Can you work these out from the model? Positions are in its coordinate system, mm. Face numbers are marked on the shaded views. A direction names the side the tool comes from. Give positions to 0.01 mm unless a question says otherwise; leave off trailing zeros. Order: outer loops, then holes, each group sorted by start corner. A loop starts at its lowest first (then second) coordinate and runs counter-clockwise, first axis right, second up. Notation, with made-up numbers: (-24.5, 67) -> (11.5, 67) arc R9 ccw to (11.5, 82) -> close; hole circle Ø5 at (-16.75, 70). An arc over 180 degrees is marked (long way). Answer as a JSON object with one key per item and string values.
```python
from build123d import *

# Parameters (mm, degrees)
F1_DEPTH       = 22.5
F3_DEPTH       = 10
F5_D           = 10
F5_CBORE_D     = 20
F5_CBORE_DEPTH = 5


with BuildPart() as f1:
    # F0 (on Front) → F1 (new body, symmetric)
    with BuildSketch(Plane.XZ):
        Polygon((0, 45), (0, 0), (65, 0), (65, 10), (55, 10), (55, 45), align=None)
    extrude(amount=F1_DEPTH, both=True)

    # F2 (on face) → F3 (cut)
    with BuildSketch(Plane.YZ.offset(55)):
        Polygon((-22.5, 45), (-22.5, 30), (22.5, 45), align=None)
    extrude(amount=-F3_DEPTH, mode=Mode.SUBTRACT)

    # F5 (through all)
    with Locations(Plane.XY.offset(45)):
        with Locations((22.5, 0)):
            CounterBoreHole(F5_D / 2, F5_CBORE_D / 2, F5_CBORE_DEPTH)


solid = f1.part
```
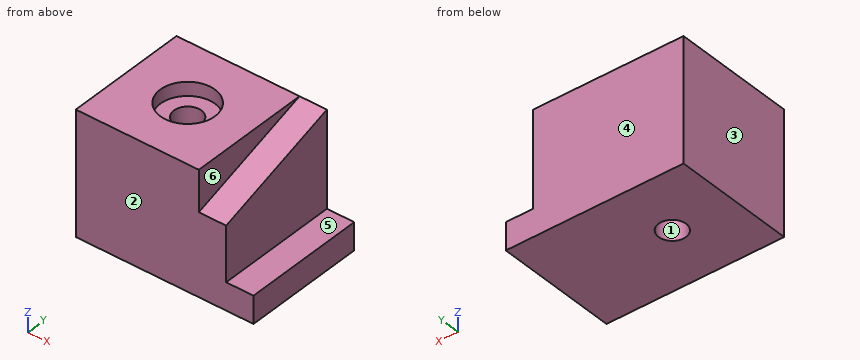
1. If we section it at D-D on z = 32: Please give me the cut outline in (x, y), then the cut area to 3 significant figures.
Worked answers:
{"outline": "(0, -22.5) -> (45, -22.5) -> (45, -16.5) -> (55, -16.5) -> (55, 22.5) -> (0, 22.5) -> close; hole circle Ø10 at (22.5, 0)", "area": "2,340 mm²"}
2. If we section it at A-A on y = 0: Please give me the cut outline in (x, z), then the cut area to 3 significant figures.
Worked answers:
{"outline": "(0, 0) -> (17.5, 0) -> (17.5, 40) -> (12.5, 40) -> (12.5, 45) -> (0, 45) -> close; (27.5, 0) -> (65, 0) -> (65, 10) -> (55, 10) -> (55, 37.5) -> (45, 37.5) -> (45, 45) -> (32.5, 45) -> (32.5, 40) -> (27.5, 40) -> close", "area": "2,000 mm²"}
3. For the marked faces 4, 5 and 6, which set-ups out of +Z, -Z, +X, -X, +Y, -Y let a thin tool reach every point of the face, with its end or its side?
Worked answers:
{"face 4": "+Z, -Z, +X, -X, +Y", "face 5": "+Z, +X, +Y, -Y", "face 6": "+Z, +X, -Y"}
4. If we section it at B-B on x = 22.5: Please give me the cut outline in (y, z).
Worked answers:
{"outline": "(-22.5, 0) -> (-5, 0) -> (-5, 40) -> (-10, 40) -> (-10, 45) -> (-22.5, 45) -> close; (5, 0) -> (22.5, 0) -> (22.5, 45) -> (10, 45) -> (10, 40) -> (5, 40) -> close"}
5. Will these pins go through, and if not, where does the flat tip stop? pin 1 Ø23 at (x, y) = (22.5, 0) entering from +Z; pin 2 Ø7.5 at (y, z) = (4, 35) entering from +X; pin 3 Ø11 at (x, y) = (61, -8.5) entering from +Z.
Worked answers:
{"pin 1": "z = 45", "pin 2": "x = 55", "pin 3": "z = 10"}
6. If we section it at C-C on z = 4.5: Please give me the cut outline in (x, y).
Worked answers:
{"outline": "(0, -22.5) -> (65, -22.5) -> (65, 22.5) -> (0, 22.5) -> close; hole circle Ø10 at (22.5, 0)"}
7. Please list where these lines run through material, in increasing order: L1, parallel to Y at x = 22.5, z = 43.3; L2, parallel to Y at x = 22.5, z = 17; L3, parallel to X at y = -7, z = 20.
Worked answers:
{"L1": "-22.5 to -10, 10 to 22.5", "L2": "-22.5 to -5, 5 to 22.5", "L3": "0 to 55"}
8. If we mould it in two halves opening along X, with no side actions, what happens to the marked faces 1, 2 and 3? For each: +X half, -X half, draft (parallel to the pull), parting line (faces both ways), or undercut.
Worked answers:
{"face 1": "undercut", "face 2": "draft", "face 3": "-X half"}
